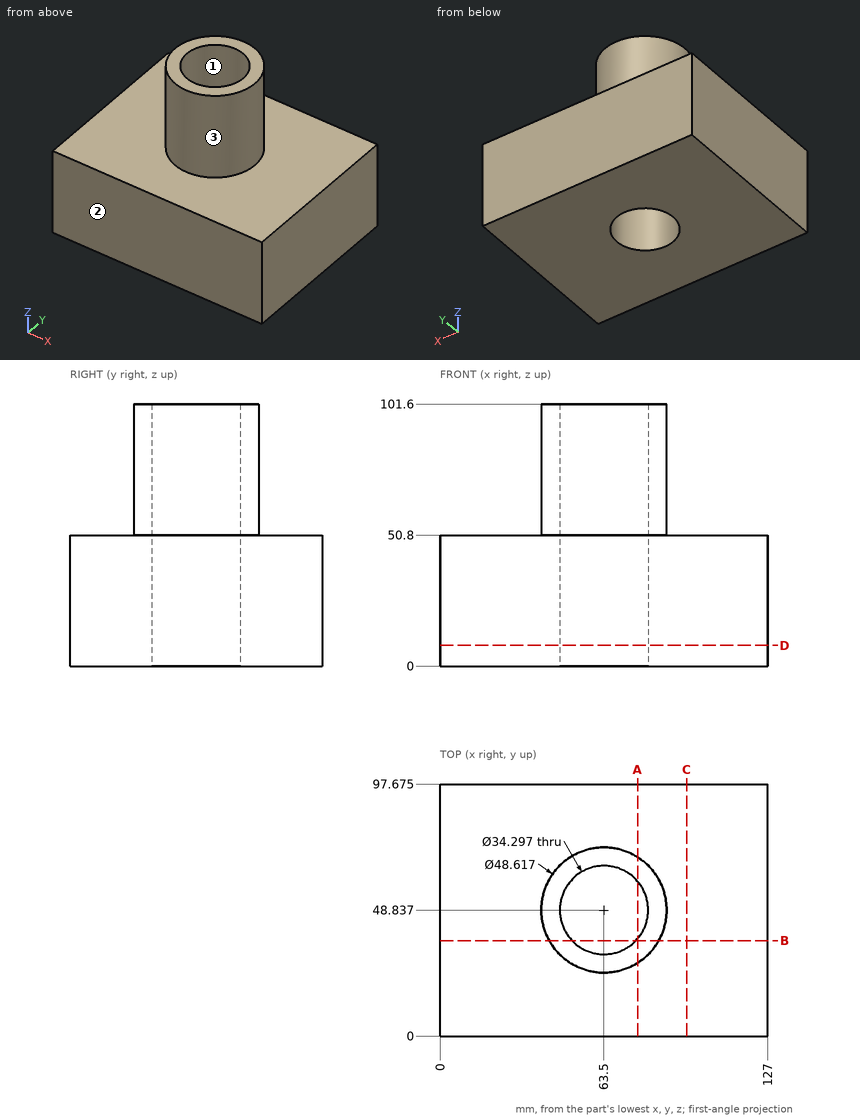
Answer from the drawing. Dimensions are ordinates in mm from the lowest x, y and z of the part. Coordinates: 2 decimals unless noted, no trailing zeros. Loops run counter-clockwise (first coordinate to the right, second up) from the corner with the lowest first, then second, coordinate; pieces in that order, holes last. Notation, with made-up numbers: (78.5, 43) - (127.5, 43) arc R26 ccw to (127.5, 81) - close; hole circle Ø5 at (80, -34). An arc over 180 degrees is marked (long way). Answer in a Markdown table with one row per item.
1. Find section D-D, the plane z = 8. Write down the section's boundary in (x, y) (1 decimal), then the cut area to 3 significant figures.
Conclusion:
| item | result |
|---|---|
| outline | (0, 0) - (127, 0) - (127, 97.7) - (0, 97.7) - close; hole circle Ø34.3 at (63.5, 48.8) |
| area | 11,500 mm² |
2. Determine the mould class of the marked faces 1, 2 and 3 for opening direction X: +X half, -X half, draft (parallel to the pull), parting line (faces both ways), or undercut.
Conclusion:
| item | result |
|---|---|
| face 1 | undercut |
| face 2 | draft |
| face 3 | parting line |
3. Find section C-C, the plane x = 95.5. Write down the section's boundary in (y, z) (1 decimal), then the cut area to 3 significant figures.
Conclusion:
| item | result |
|---|---|
| outline | (0, 0) - (97.7, 0) - (97.7, 50.8) - (0, 50.8) - close |
| area | 4,960 mm² |
4. Straight lines are drawn through the part: line 1 (Z direction, x = 10, y = 52.5); line 2 (Y direction, x = 53, z = 36) (1 decimal); line 3 (X direction, y = 57, z = 89) (1 decimal). For each, find the intervals that lie inside material, in ascending order.
Conclusion:
| item | result |
|---|---|
| line 1 | z = 0 to 50.8 |
| line 2 | y = 0 to 35.3, 62.4 to 97.7 |
| line 3 | x = 40.6 to 48.4, 78.6 to 86.4 |
5. Find section B-B, the plane y = 37. Write down the section's boundary in (x, z).
Conclusion:
| item | result |
|---|---|
| outline | (0, 0) - (51.09, 0) - (51.09, 101.6) - (42.27, 101.6) - (42.27, 50.8) - (0, 50.8) - close; (75.91, 0) - (127, 0) - (127, 50.8) - (84.73, 50.8) - (84.73, 101.6) - (75.91, 101.6) - close |
6. Given pin 1 (4 mm diameter, centred on x = 26.5, y = 67.5, fed in from +Z); pin 2 (1 mm diameter, centred on x = 75.5, z = 72.5, fed in from -Y), each flat-ended and moving along its own axis, determine where each tip first touches the part or whether it passes through.
Conclusion:
| item | result |
|---|---|
| pin 1 | stops at z = 50.8 |
| pin 2 | stops at y = 27.42 |
7. Find section A-A, the plane x = 76.5. Write down the section's boundary in (y, z) (1 decimal), then the cut area to 3 significant figures.
Conclusion:
| item | result |
|---|---|
| outline | (0, 0) - (37.7, 0) - (37.7, 101.6) - (28.3, 101.6) - (28.3, 50.8) - (0, 50.8) - close; (60, 0) - (97.7, 0) - (97.7, 50.8) - (69.4, 50.8) - (69.4, 101.6) - (60, 101.6) - close |
| area | 4,780 mm² |
